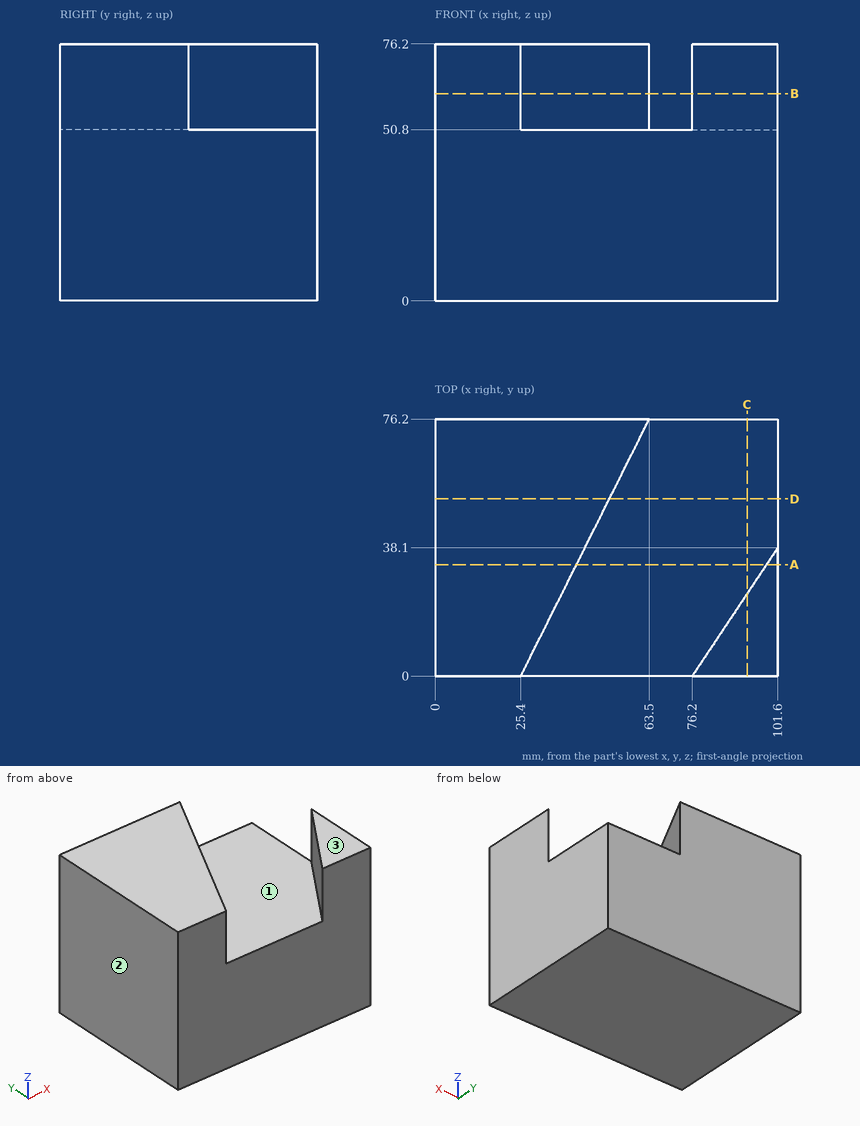
Input: dimensioned drawing with shaded views. Units: mm. Origin: part minimum x, y, z. Give positions to 0.01 mm unless a question says otherwise; leave off trailing zeros. Write each loop counter-clockwise with the first axis right and the second up, starting at its lowest first coordinate (ties: lowest second). Pieces come first, ordered by that corner, then holes.
1. Section query D-D (y = 52.5). Return the cut outline in (x, z), then the cut area to 3 significant figures.
2. Pull-direction query (X, two-part tool) for the marked faces 1, 2 and 3; classes: +X half, -X half, draft (parallel to the pull), parting line (faces both ways), or undercut.
3. Section query B-B (z = 61.5). Return the cut outline in (x, y), then the cut area to 3 significant figures.
4. Section query C-C (x = 92.5). Return the cut outline in (y, z).
5. Material intervals for line 1 along Z through (x, y) = (77.5, 59.5); line 2 along X through (y, z) = (9, 64); line 3 along Y through (x, z) = (30, 53), sorted ascending.
6. First-contact query: pin 1 (4 mm diameter, centred on x = 42.5, y = 27, fed in from +Z). Flat tip, straight axial feed; report the tip coordinate or a pass-through.
7. Section query A-A (y = 33). Return the cut outline in (x, z).
Output values:
1. outline: (0, 0) - (101.6, 0) - (101.6, 50.8) - (51.65, 50.8) - (51.65, 76.2) - (0, 76.2) - close
1. area: 6,470 mm2
2. face 1: undercut
2. face 2: -X half
2. face 3: draft
3. outline: (0, 0) - (25.4, 0) - (63.5, 76.2) - (0, 76.2) - close; (76.2, 0) - (101.6, 0) - (101.6, 38.1) - close
3. area: 3,870 mm2
4. outline: (0, 0) - (76.2, 0) - (76.2, 50.8) - (24.45, 50.8) - (24.45, 76.2) - (0, 76.2) - close
5. line 1: z = 0 to 50.8
5. line 2: x = 0 to 29.9, 82.2 to 101.6
5. line 3: y = 9.2 to 76.2
6. pin 1: stops at z = 50.8
7. outline: (0, 0) - (101.6, 0) - (101.6, 76.2) - (98.2, 76.2) - (98.2, 50.8) - (41.9, 50.8) - (41.9, 76.2) - (0, 76.2) - close
